Could you check a few things on this model? Use its own coordinates, in mm. Face numbers are marked on the shaded views. A direction names the side the tool comes from. Round coordinates to 2 decimals unless told otherwise and drop trailing zeros. Loops run counter-clockwise (first coordinate to the right, second up) from the corner with the lowest first, then second, coordinate; pieces in that order, holes last. Notation, with made-up numbers: M 26,-27 L 35,-27 A34 cw 35,3 Z; hole C -14.5,38 d6. An arc over 180 degrees is marked long. Return JSON: item names as keys, results as strings. Group by question number.
```python
from build123d import *

# Parameters (mm, degrees)
SKETCH_1_R                   = 4
EXTRUDE_1_DEPTH              = 30
HOLE_WIZARD_M5_1_D           = 4.2
HOLE_WIZARD_M5_1_DEPTH       = 18
HOLE_WIZARD_M5_1_CSINK_D     = 5.05
HOLE_WIZARD_M5_1_CSINK_ANGLE = 90
HOLE_WIZARD_M5_1_TIP         = 1.2618073
SKETCH_4_R                   = 2.15
CUT_EXTRUDE_1_DEPTH          = 30


with BuildPart() as part:
    # 草图1 → 凸台-拉伸1 (new body)
    with BuildSketch(Plane.XY):
        Polygon((-5, 11), (5, 11), (8, 7), (15, 7), (15, -3), (17, -5), (17, -11), (7, -11), (6, -10), (-6, -10), (-7, -11), (-17, -11), (-17, -5), (-15, -3), (-15, 7), (-8, 7), align=None)
        Circle(SKETCH_1_R, mode=Mode.SUBTRACT)
    extrude(amount=EXTRUDE_1_DEPTH)

    # M5 螺纹孔1
    with Locations(Plane(origin=(0, -11, 0), x_dir=(-1, 0, 0), z_dir=(0, -1, 0))):
        with Locations((12, -24), (12, -6), (-12, -24), (-12, -6)):
            CounterSinkHole(HOLE_WIZARD_M5_1_D / 2, HOLE_WIZARD_M5_1_CSINK_D / 2, depth=HOLE_WIZARD_M5_1_DEPTH, counter_sink_angle=HOLE_WIZARD_M5_1_CSINK_ANGLE)
            with Locations((0, 0, -(HOLE_WIZARD_M5_1_DEPTH + HOLE_WIZARD_M5_1_TIP / 2))):  # 118° drill point
                Cone(0, HOLE_WIZARD_M5_1_D / 2, HOLE_WIZARD_M5_1_TIP, mode=Mode.SUBTRACT)

    # 草图4 → 切除-拉伸1 (cut)
    with BuildSketch(Plane.XZ.offset(11)):
        with Locations((-12, 24)):
            Circle(SKETCH_4_R)
        with Locations(Location((12, 24, 0), (0, 0, 270))):
            Circle(SKETCH_4_R)
        with Locations(Location((12, 6, 0), (0, 0, 270))):
            Circle(SKETCH_4_R)
        with Locations((-12, 6)):
            Circle(SKETCH_4_R)
    extrude(amount=-CUT_EXTRUDE_1_DEPTH, mode=Mode.SUBTRACT)


solid = part.part
```
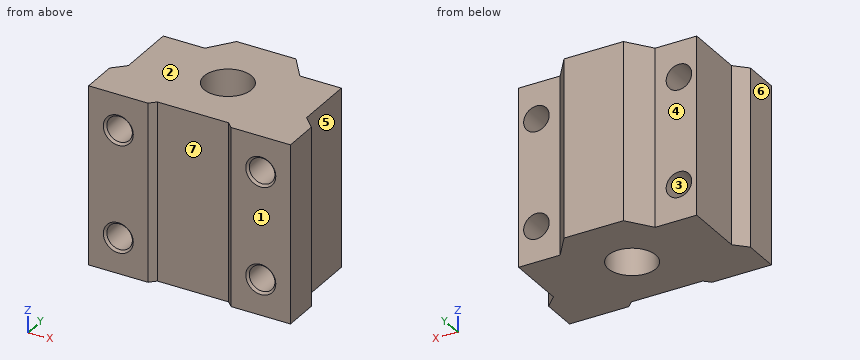
1. If we section it at D-D, the plane y = 5.75: Please give me the cut outline in (x, z), then the cut area to 3 significant figures.
2. If we section it at B-B, the plane y = -1.75: Please give me the cut outline in (x, z).
3. We'd pull the mould along Z, two halves only. Please class the marked faces 1, 2 and 3: +Z half, -Z half, draft (parallel to the pull), parting line (faces both ways), or undercut.
4. On a 3-axis mill with a long thin cutter (end or side, diameter ignored), from which of +Z, -Z, +X, -X, +Y, -Y can I reach the whole of each face in a straight line? I mean the marked faces 4, 5, 6 and 7. Say none if no direction works.
5. I'm going to push flat-ended pins straight in: pin 1 Ø8 at (x, y) = (-8, 6) entering from -Z; pin 2 Ø1.5 at (y, z) = (-2.5, 13) entering from -X; pin 3 Ø5.5 at (x, z) = (-11.5, 11) entering from +Y; pin 4 Ø8 at (y, z) = (1.5, 20) entering from +X. Where does each tip first touch, or does it pass through?
6. I need wall thicknesses on probe 1 along Z at (x, y) = (-12, 0.75); probe 2 along X at (y, z) = (-2.75, 23); probe 3 along Y at (x, z) = (0, 8.75). Which ranges of each line are inside material? Lowest first, please.
7. If we section it at C-C, the plane x = 0: Please give me the cut outline in (y, z), then the cut area to 3 significant figures.
8. If we section it at A-A, the plane z = 6: Give the number of separate pieces and of enclosed holes in the cut face, then the cut area to 3 significant figures.
Geometry results:
{
 "1": {"outline": "M -15,0 L 15,0 L 15,30 L -15,30 Z; hole C -12,6 d4.3; hole C -12,24 d4.3; hole C 12,6 d4.3; hole C 12,24 d4.3", "area": "842 mm^2"},
 "2": {"outline": "M -15,0 L -3.6,0 L -3.6,30 L -15,30 Z; M 3.6,0 L 15,0 L 15,30 L 3.6,30 Z; hole C -12,6 d4.3; hole C -12,24 d4.3; hole C 12,6 d4.3; hole C 12,24 d4.3"},
 "3": {"face 1": "draft", "face 2": "+Z half", "face 3": "undercut"},
 "4": {"face 4": "+Z, -Z, -X, +Y", "face 5": "+Z, -Z, +X, +Y", "face 6": "+Z, -Z, -X, +Y, -Y", "face 7": "+Z, -Z, -Y"},
 "5": {"pin 1": "z = 0", "pin 2": "x = -15.25", "pin 3": "y = 7", "pin 4": "x = 15"},
 "6": {"probe 1": "0 to 3.85, 8.15 to 21.85, 26.15 to 30", "probe 2": "-15 to -13.9, -10.1 to -2.9, 2.9 to 10.1, 13.9 to 15", "probe 3": "-10 to -4, 4 to 11"},
 "7": {"outline": "M -10,0 L -4,0 L -4,30 L -10,30 Z; M 4,0 L 11,0 L 11,30 L 4,30 Z", "area": "390 mm^2"},
 "8": {"separate pieces": "3", "enclosed holes": "1", "area": "402 mm^2"}
}
